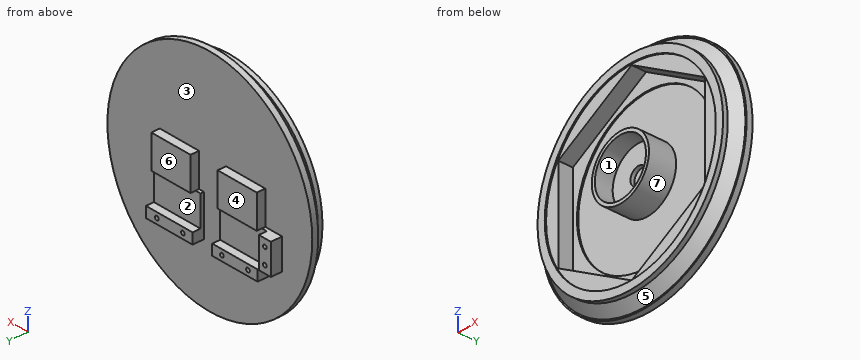
```python
from build123d import *

# Parameters (mm, degrees)
SKETCH2_R           = 71
BOSS_EXTRUDE1_DEPTH = 11
SKETCH10_W          = 37.65
SKETCH10_H          = 8
SKETCH10_R          = 1.5
SKETCH10_W_2        = 10
SKETCH10_H_2        = 23
SKETCH10_W_3        = 1
BOSS_EXTRUDE6_DEPTH = 8.5
SKETCH12_R          = 57.5
SKETCH12_R_2        = 23.75
CUT_EXTRUDE8_DEPTH  = 1
SKETCH11_W          = 38.65
SKETCH11_H          = 23
BOSS_EXTRUDE7_DEPTH = 2.5
SKETCH14_W          = 32.5
SKETCH14_H          = 25
BOSS_EXTRUDE8_DEPTH = 6.4


with BuildPart() as part:
    # Sketch1 → Revolve1 (revolve)
    with BuildSketch(Plane.XY, mode=Mode.PRIVATE) as revolve1_sk:
        Polygon((0, 12), (0, 15), (85, 15), (85, 10.5), (84, 10.5), (77, 3.5), (77, 0), (71, 0), (71, 12), (23.75, 12), (23.75, -7.5), (21.25, -7.5), (21.25, 6), (6.5, 6), (6.5, 9), (0, 9), align=None)
    revolve(revolve1_sk.sketch.rotate(Axis((0, 12, 0), (0, -1, 0)), 180), axis=Axis((0, 12, 0), (0, -1, 0)))

    # Sketch2 → Boss-Extrude1 (add)
    with BuildSketch(Plane.XZ.offset(-12)):
        with Locations(Location((0, 0, 0), (0, 0, 180))):
            Circle(SKETCH2_R)
        Polygon((0, 70.292395274), (-60.875, 35.146197637), (-60.875, -35.146197637), (0, -70.292395274), (60.875, -35.146197637), (60.875, 35.146197637), align=None, mode=Mode.SUBTRACT)
    extrude(amount=BOSS_EXTRUDE1_DEPTH)

    # Sketch10 → Boss-Extrude6 (add)
    # profile 1 of 4: a face of its own
    with BuildSketch(Plane(origin=(0, 15, 0), x_dir=(1, 0, 0), z_dir=(0, 1, 0))):
        with Locations((-30.175, 36)):
            Rectangle(SKETCH10_W, SKETCH10_H)
        with Locations(Location((-41, 36, 0), (0, 0, 180))):
            Circle(SKETCH10_R, mode=Mode.SUBTRACT)
        with Locations(Location((-19.35, 36, 0), (0, 0, 180))):
            Circle(SKETCH10_R, mode=Mode.SUBTRACT)
    # profile 2 of 4: a face of its own
    with BuildSketch(Plane(origin=(0, 15, 0), x_dir=(1, 0, 0), z_dir=(0, 1, 0))):
        with Locations((-55, 20.5)):
            Rectangle(SKETCH10_W_2, SKETCH10_H_2)
        with Locations(Location((-55, 14.5, 0), (0, 0, 180))):
            Circle(SKETCH10_R, mode=Mode.SUBTRACT)
        with Locations(Location((-55, 26.5, 0), (0, 0, 180))):
            Circle(SKETCH10_R, mode=Mode.SUBTRACT)
    # profile 3 of 4: a face of its own
    with BuildSketch(Plane(origin=(0, 15, 0), x_dir=(1, 0, 0), z_dir=(0, 1, 0))):
        with Locations((23.825, 36)):
            Rectangle(SKETCH10_W, SKETCH10_H)
        with Locations(Location((13, 36, 0), (0, 0, 180))):
            Circle(SKETCH10_R, mode=Mode.SUBTRACT)
        with Locations(Location((34.65, 36, 0), (0, 0, 180))):
            Circle(SKETCH10_R, mode=Mode.SUBTRACT)
    # profile 4 of 4: a face of its own
    with BuildSketch(Plane(origin=(0, 15, 0), x_dir=(1, 0, 0), z_dir=(0, 1, 0))):
        with Locations((43.15, 36)):
            Rectangle(SKETCH10_W_3, SKETCH10_H)
    extrude(amount=BOSS_EXTRUDE6_DEPTH)

    # Sketch12 → Cut-Extrude8 (cut)
    with BuildSketch(Plane.XZ.offset(-12)):
        Circle(SKETCH12_R)
        with Locations(Location((0, 0, 0), (0, 0, 180))):
            Circle(SKETCH12_R_2, mode=Mode.SUBTRACT)
    extrude(amount=-CUT_EXTRUDE8_DEPTH, mode=Mode.SUBTRACT)

    # Sketch11 → Boss-Extrude7 (add)
    with BuildSketch(Plane(origin=(0, 15, 0), x_dir=(1, 0, 0), z_dir=(0, 1, 0))):
        with Locations((-30.675, 20.5)):
            Rectangle(SKETCH11_W, SKETCH11_H)
        with Locations((24.325, 20.5)):
            Rectangle(SKETCH11_W, SKETCH11_H)
    extrude(amount=BOSS_EXTRUDE7_DEPTH)

    # Sketch14 → Boss-Extrude8 (add)
    with BuildSketch(Plane(origin=(0, 15, 0), x_dir=(1, 0, 0), z_dir=(0, 1, 0))):
        with Locations((-29.75, -3.5)):
            Rectangle(SKETCH14_W, SKETCH14_H)
        with Locations((25.25, -3.5)):
            Rectangle(SKETCH14_W, SKETCH14_H)
    extrude(amount=BOSS_EXTRUDE8_DEPTH)


solid = part.part
```
The listing builds one solid part. Answer for the finished solid, in the listing's coordinates (mm). Face numbers are marked on the shaded views. A direction names the side the tool comes from. Coordinates: 2 decimals unless noted, no trailing zeros. Write each loop counter-clockwise with the first axis right and the second up, starting at its lowest first coordinate (ties: lowest second). Pieces come first, ordered by that corner, then holes.
Q1. Find the intervals of material crossed by line 1 along Z through (x, y) = (-55, 18.75); line 2 along Z through (x, y) = (0, 12.7); line 3 along Z through (x, y) = (0, 0.3), in increasing order.
Returned:
line 1: z = -32 to -28, -25 to -16, -13 to -9
line 2: z = -85 to -57.5, -23.75 to 23.75, 57.5 to 85
line 3: z = -77 to -71, -23.75 to -21.25, 21.25 to 23.75, 71 to 77
Q2. Given P1, Ø3, axis at x = 8.5, y = -3.5, coming from the +Z side (3 decimals); P2, Ø3, axis at y = 17.5, z = 8.5, coming from the +X side; P3, Ø6, axis at y = 19, z = 2.5, coming from the -X side, each flat-ended and moving along its own axis, determine where each tip first touches the part or whether it passes through.
Returned:
P1: stops at z = 22.695
P2: stops at x = 41.5
P3: stops at x = -46
Q3. Section A-A, the plane y = -3 is taken. Write down the section's boundary in (x, z), then the cut area to 3 significant figures.
Returned:
outline: circle Ø47.5 at (0, 0); hole circle Ø42.5 at (0, 0)
area: 353 mm2
Q4. Which of the six approach directions +Z, -Z, +X, -X, +Y, -Y give full straight-line access (tool end or side, diameter ignored) to the marked faces 1, 2, 3 and 4?
Returned:
face 1: -Y
face 2: +X, +Y
face 3: +Y
face 4: +Z, +X, -X, +Y
Q5. The mould has two halves that part along Z. Classify the marked faces 5, 6 and 7: released by +Z, released by -Z, zero draft, split by the parting line, or undercut.
Returned:
face 5: split by the parting line
face 6: zero draft
face 7: undercut
